Design review of the part built by this model. Coordinates are the model's own, in mm. A direction names the side the tool comes from. Give positions to 0.01 mm unless a question says otherwise; leave off trailing zeros. Write each loop counter-clockwise with the first axis right and the second up, starting at its lowest first coordinate (ties: lowest second). Pieces come first, ordered by that corner, then holes.
```python
from build123d import *

# Parameters (mm, degrees)
F1_R     = 3.228028
F1_R_2   = 3.012468
F2_DEPTH = 6.35


with BuildPart() as f2:
    # F1 (on face) → F2 (new body)
    with BuildSketch(Plane.XY):
        with BuildLine():
            ThreePointArc((-91.947787, 87.109275), (-85.086599, 93.970463), (-91.947787, 100.83165))
            Line((-91.947787, 100.83165), (-99.291265, 100.83165))
            Line((-99.291265, 100.83165), (-99.291265, 108.071581))
            Line((-99.291265, 108.071581), (-101.831265, 108.071581))
            Line((-101.831265, 108.071581), (-101.831265, 67.195773))
            Line((-101.831265, 67.195773), (-86.591265, 67.195773))
            Line((-86.591265, 67.195773), (-86.591265, 74.484758))
            Line((-86.591265, 74.484758), (-83.508379, 74.484758))
            Line((-83.508379, 74.484758), (-83.508379, 77.024758))
            Line((-83.508379, 77.024758), (-89.131265, 77.024758))
            Line((-89.131265, 77.024758), (-89.131265, 69.735773))
            Line((-89.131265, 69.735773), (-99.291265, 69.735773))
            Line((-99.291265, 69.735773), (-99.291265, 87.109275))
            Line((-99.291265, 87.109275), (-91.947787, 87.109275))
        make_face()
        with Locations((-91.947787, 93.970463)):
            Circle(F1_R, mode=Mode.SUBTRACT)
        with BuildLine():
            Line((-76.610117, 77.024758), (-83.508379, 77.024758))
            Line((-83.508379, 77.024758), (-83.508379, 74.484758))
            Line((-83.508379, 74.484758), (-79.150117, 74.484758))
            Line((-79.150117, 74.484758), (-79.150117, 67.417324))
            Line((-79.150117, 67.417324), (-2.54, 67.417324))
            Line((-2.54, 67.417324), (-2.54, 61.251126))
            Line((-2.54, 61.251126), (103.91023, 61.251126))
            Line((103.91023, 61.251126), (106.528006, 56.480713))
            Line((106.528006, 56.480713), (136.366479, 56.480713))
            Line((136.366479, 56.480713), (138.906479, 59.101462))
            Line((138.906479, 59.101462), (138.906479, 108.071581))
            Line((138.906479, 108.071581), (136.366479, 108.071581))
            Line((136.366479, 108.071581), (136.366479, 85.211581))
            Line((136.366479, 85.211581), (128.938311, 85.211581))
            Line((128.938311, 85.211581), (128.938311, 69.971581))
            ThreePointArc((128.938311, 69.971581), (124.35225, 68.268028), (122.379587, 63.791126))
            Line((122.379587, 63.791126), (104.599587, 63.791126))
            Line((104.599587, 63.791126), (0, 63.791126))
            Line((0, 63.791126), (0, 69.957324))
            Line((0, 69.957324), (-76.610117, 69.957324))
            Line((-76.610117, 69.957324), (-76.610117, 77.024758))
        make_face()
        with Locations((130.075902, 61.770894)):
            Circle(F1_R_2, mode=Mode.SUBTRACT)
    extrude(amount=F2_DEPTH)


solid = f2.part
```
(1) Consider section C-C, the plane x = -46. Give the boundary of the cut face in (y, z), then the cut area to 3 significant figures.
Resolved:
outline: (67.42, 0) - (69.96, 0) - (69.96, 6.35) - (67.42, 6.35) - close
area: 16.1 mm2
(2) Clearance check with flat-ended pins moving along their axes: P1, Ø3, axis at x = -51.5, z = 3.5, coming from the +Y side; P2, Ø1.9, axis at x = -81.5, z = 2.5, coming from the -Y side; P3, Ø1.9, axis at x = -94.5, z = 2, coming from the +Y side. State where each tip first meets the part, or that it passes through.
Resolved:
P1: stops at y = 69.96
P2: stops at y = 74.48
P3: stops at y = 100.83
(3) To check wall thickness, follow L1, parallel to X at y = 94, z = 3.5; L2, parallel to X at y = 94.5, z = 2; L3, parallel to X at y = 83, z = 1.75. State the ranges of each line that lie inside material, in increasing order.
Resolved:
L1: x = -101.83 to -95.18, -88.72 to -85.09, 136.37 to 138.91
L2: x = -101.83 to -95.13, -88.76 to -85.11, 136.37 to 138.91
L3: x = -101.83 to -99.29, 128.94 to 138.91
(4) Mouldability with a two-part tool opening along X and no side actions: class faces 1 (the face through (36, 63, 0)), 2 (the face through (-99.291, 78, 3)), 3 (the face through (138.906, 83, 3)) as pulls with the +X half, pulls with the -X half, needs draft (parallel to the pull), parting line crosses it, or undercut.
Resolved:
face 1: needs draft
face 2: undercut
face 3: pulls with the +X half
(5) Consider section A-A, the plane y = 79. Give the boundary of the cut face in (x, z).
Resolved:
outline: (-101.83, 0) - (-99.29, 0) - (-99.29, 6.35) - (-101.83, 6.35) - close; (128.94, 0) - (138.91, 0) - (138.91, 6.35) - (128.94, 6.35) - close
(6) Consider section D-D, the plane x = 115. Give the boundary of the cut face in (y, z), then the cut area to 3 significant figures.
Resolved:
outline: (56.48, 0) - (63.79, 0) - (63.79, 6.35) - (56.48, 6.35) - close
area: 46.4 mm2
(7) Tool access review of faces 4 (the face through (62, 63.791, 3)), 5 (the face through (-85.09, 93.82, 3.13)), 6 (the face through (-83, 74.485, 3)): name each direction out of +Z, -Z, +X, -X, +Y, -Y from which nothing blocks a thin tool from reaching the whole face with its end or side.
Resolved:
face 4: +Z, -Z, +Y
face 5: +Z, -Z
face 6: +Z, -Z, -Y
(8) Consider section B-B, the plane z = 5.25. Give the number of separate pieces and of enclosed holes in the cut face, then the cut area to 3 significant figures.
Resolved:
separate pieces: 1
enclosed holes: 2
area: 1,340 mm2
